Job drawing, mm, ordinate dimensions from the low corner. One solid piece. A direction names the side the tool comes from. Coordinates: 2 decimals unless noted, no trailing zeros. Loops run counter-clockwise (first coordinate to the right, second up) from the corner with the lowest first, then second, coordinate; pieces in that order, holes last. Notation, with made-up numbers: (-13.75, -20) - (1.25, -20) arc R14 ccw to (1.25, 2) - close; hole circle Ø11 at (86, -10). An arc over 180 degrees is marked (long way). Use a Markdown table: item, result. Add a question column.
1. 3-axis set-ups, long thin cutter, end or side, ignore diameter. For the marked faces 1 and 2: which of +Z, -Z, +X, -X, +Y, -Y reach the whole face in a straight line?
2. Band-saw the part on B-B, the plane x = 6.35. Give the cut face in (y, z) (3 decimals).
3. Wall check: probe 1 along Z at (x, y) = (1, 1.6) (3 decimals); probe 2 along Z at (x, y) = (8.25, 1.4) (3 decimals). Give the ranges that are in metal, low to high. Write a range as [from, to].
4. Band-saw the part on C-C, the plane z = 6.35. Give the cut face in (x, y) (3 decimals), plus the area to 3 significant figures.
5. Band-saw the part on A-A, the plane y = 0.5. Give the cut face in (x, z) (3 decimals), plus the area to 3 significant figures.
6. Pull direction X, two halves, no side cores. Call the marked faces 3, 4 and 5: pulls with the +X half, pulls with the -X half, needs draft (parallel to the pull), parting line crosses it, or undercut.
7. Band-saw the part on D-D, the plane z = 3.5. Give the cut face in (x, y) (3 decimals).
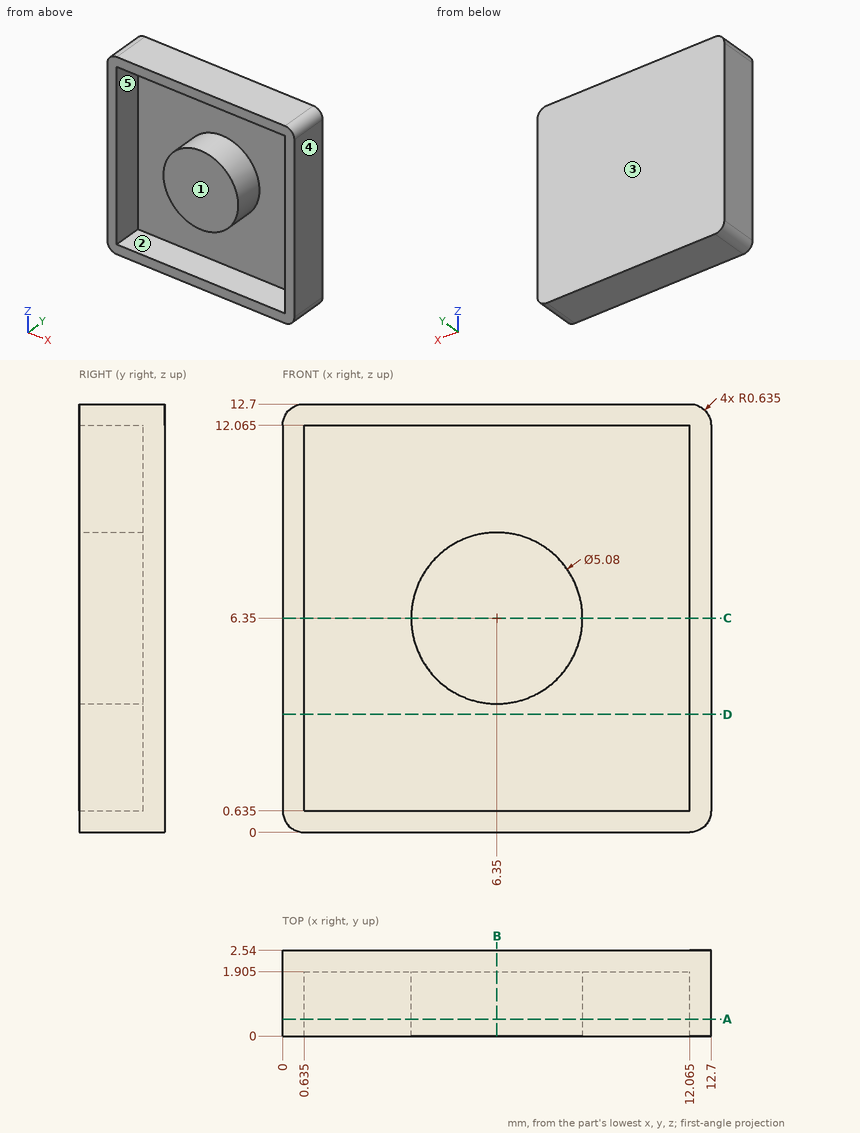
Geometry check:
| question | item | result |
|---|---|---|
| 1 | face 1 | +Z, -Z, +X, -X, -Y |
| 1 | face 2 | -Y |
| 2 | outline | (0, 0) - (2.54, 0) - (2.54, 12.7) - (0, 12.7) - (0, 12.065) - (1.905, 12.065) - (1.905, 8.89) - (0, 8.89) - (0, 3.81) - (1.905, 3.81) - (1.905, 0.635) - (0, 0.635) - close |
| 3 | probe 1 | z = [0, 0.635], [12.065, 12.7] |
| 3 | probe 2 | z = [0, 0.635], [4.664, 8.036], [12.065, 12.7] |
| 4 | outline | (0, 0) - (0.635, 0) - (0.635, 1.905) - (3.81, 1.905) - (3.81, 0) - (8.89, 0) - (8.89, 1.905) - (12.065, 1.905) - (12.065, 0) - (12.7, 0) - (12.7, 2.54) - (0, 2.54) - close |
| 4 | area | 20.2 mm^2 |
| 5 | outline | (0, 0.635) arc R0.635 ccw to (0.635, 0) - (12.065, 0) arc R0.635 ccw to (12.7, 0.635) - (12.7, 12.065) arc R0.635 ccw to (12.065, 12.7) - (0.635, 12.7) arc R0.635 ccw to (0, 12.065) - close; circle Ø5.08 at (6.35, 6.35); hole (0.635, 0.635) - (12.065, 0.635) - (12.065, 12.065) - (0.635, 12.065) - close |
| 5 | area | 50.6 mm^2 |
| 6 | face 3 | needs draft |
| 6 | face 4 | pulls with the +X half |
| 6 | face 5 | undercut |
| 7 | outline | (0, 0) - (0.635, 0) - (0.635, 1.905) - (12.065, 1.905) - (12.065, 0) - (12.7, 0) - (12.7, 2.54) - (0, 2.54) - close |
